Could you check a few things on this model? Use its own coordinates, in mm. Coordinates: 2 decimals unless noted, no trailing zeros. Order: outer loops, then holes, each group sorted by start corner. A loop starts at its lowest first (then second) coordinate and runs counter-clockwise, first axis right, second up. Notation, with made-up numbers: (82.5, 32) - (116.5, 32) arc R24 ccw to (116.5, 53) - close; hole circle Ø6 at (32.25, -27.75). An arc over 180 degrees is marked (long way). Answer as a JSON object with one key per item and string values. Group by question number.
(1) Please list where these lines run through material, in increasing order: probe 1 along Y at (x, z) = (4.5, 2.7); probe 2 along Y at (x, z) = (2.75, 2.7); probe 3 along X at (y, z) = (270, 0.75).
(2) Will this pin go through, and if not, where does the flat tip stop? P1, Ø4, axis at x = 4, y = 270, coming from the -Z side.
(3) Imagine slicing it at B-B, the plane x = 4. Write out the boundary of the cut face in (y, z), and give its area (3 significant figures).
(4) Imagine slicing it at A-A, the plane z = 2.05. Write out the boundary of the cut face in (x, y), and give its area (3 significant figures).
from build123d import *

# Parameters (mm, degrees)
ESQUISSE1_W             = 8
ESQUISSE1_H             = 300
BOSS_EXTRU_1_DEPTH      = 3
ESQUISSE2_R             = 2.25
ENL_V_MAT_EXTRU_1_DEPTH = 301.121642005
ESQUISSE4_W             = 3
ESQUISSE4_H             = 300
BOSS_EXTRU_2_DEPTH      = 3


with BuildPart() as part:
    # Esquisse1 → Boss.-Extru.1 (new body)
    with BuildSketch(Plane.XY):
        with Locations((4, 150)):
            Rectangle(ESQUISSE1_W, ESQUISSE1_H)
    extrude(amount=BOSS_EXTRU_1_DEPTH)

    # Esquisse2 → Enlèv. mat.-Extru.1 (cut, through all)
    with BuildSketch(Plane.XY.offset(3)):
        with Locations((4, 110)):
            Circle(ESQUISSE2_R)
        with Locations((4, 30)):
            Circle(ESQUISSE2_R)
        with Locations(Location((4, 270, 0), (0, 0, 180))):
            Circle(ESQUISSE2_R)
        with Locations(Location((4, 190, 0), (0, 0, 180))):
            Circle(ESQUISSE2_R)
    extrude(amount=-ENL_V_MAT_EXTRU_1_DEPTH, mode=Mode.SUBTRACT)

    # Esquisse4 → Boss.-Extru.2 (add)
    with BuildSketch(Plane.XY.offset(3)):
        with Locations((9.5, 150)):
            Rectangle(ESQUISSE4_W, ESQUISSE4_H)
    extrude(amount=-BOSS_EXTRU_2_DEPTH)


solid = part.part
Result set:
{
 "1": {"probe 1": "y = 0 to 27.81, 32.19 to 107.81, 112.19 to 187.81, 192.19 to 267.81, 272.19 to 300", "probe 2": "y = 0 to 28.13, 31.87 to 108.13, 111.87 to 188.13, 191.87 to 268.13, 271.87 to 300", "probe 3": "x = 0 to 1.75, 6.25 to 11"},
 "2": {"P1": "passes through"},
 "3": {"outline": "(0, 0) - (27.75, 0) - (27.75, 3) - (0, 3) - close; (32.25, 0) - (107.75, 0) - (107.75, 3) - (32.25, 3) - close; (112.25, 0) - (187.75, 0) - (187.75, 3) - (112.25, 3) - close; (192.25, 0) - (267.75, 0) - (267.75, 3) - (192.25, 3) - close; (272.25, 0) - (300, 0) - (300, 3) - (272.25, 3) - close", "area": "846 mm^2"},
 "4": {"outline": "(0, 0) - (11, 0) - (11, 300) - (0, 300) - close; hole circle Ø4.5 at (4, 30); hole circle Ø4.5 at (4, 110); hole circle Ø4.5 at (4, 190); hole circle Ø4.5 at (4, 270)", "area": "3,240 mm^2"}
}
